from build123d import *

# Parameters (mm, degrees)
F0_R      = 174
F1_DEPTH  = 10
F2_R      = 5
F3_DEPTH  = 10
F4_R      = 5
F5_DEPTH  = 10
F6_R      = 10
F7_DEPTH  = 50
F9_R      = 9
F8_R      = 9
F10_R     = 9
F11_DEPTH = 60


with BuildPart() as f1:
    # F0 (on Top) → F1 (new body)
    with BuildSketch(Plane.XY):
        Circle(F0_R)
    extrude(amount=F1_DEPTH)

    # F2 (on face) → F3 (cut, through all)
    with BuildSketch(Plane.XY.offset(10)):
        with Locations((0, 160)):
            Circle(F2_R)
        with Locations((-113.137085, 113.137085)):
            Circle(F2_R)
        with Locations((-160, 0)):
            Circle(F2_R)
        with Locations((-113.137085, -113.137085)):
            Circle(F2_R)
        with Locations((0, -160)):
            Circle(F2_R)
        with Locations((113.137085, -113.137085)):
            Circle(F2_R)
        with Locations((160, 0)):
            Circle(F2_R)
        with Locations((113.137085, 113.137085)):
            Circle(F2_R)
    extrude(amount=-F3_DEPTH, mode=Mode.SUBTRACT)

    # F4 (on face) → F5 (cut, through all)
    with BuildSketch(Plane.XY.offset(10)):
        Circle(F4_R)
    extrude(amount=-F5_DEPTH, mode=Mode.SUBTRACT)

    # F6 (on face) → F7 (join)
    with BuildSketch(Plane.XY.offset(10)):
        with Locations((80, 0)):
            Circle(F6_R)
        with Locations((-40, 0)):
            Circle(F6_R)
        with Locations((-80, 0)):
            Circle(F6_R)
    extrude(amount=F7_DEPTH)

    # F9 (on face) + F8 (on face) + F10 (on face) → F11 (cut, through all)
    with BuildSketch(Plane.XY.offset(60)):
        with Locations((-80, 0)):
            Circle(F9_R)
    with BuildSketch(Plane.XY.offset(60)):
        with Locations((-40, 0)):
            Circle(F8_R)
    with BuildSketch(Plane.XY.offset(60)):
        with Locations((80, 0)):
            Circle(F10_R)
    extrude(amount=-F11_DEPTH, mode=Mode.SUBTRACT)


solid = f1.part
Check sheet for the modelled part. Datum: model origin and axes. Units: mm. A direction names the side the tool comes from. Round coordinates to 2 decimals unless told otherwise and drop trailing zeros. Order: outer loops, then holes, each group sorted by start corner. A loop starts at its lowest first (then second) coordinate and runs counter-clockwise, first axis right, second up. Notation, with made-up numbers: M 5,-13 L 47,-13 A22 ccw 47,16 Z; hole C -13,-9.75 d9. An arc over 180 degrees is marked long. One line per item, written item: value. Start each with the question number.
1. Section check A-A on z = 54.5. Enter the section's corners in (x, y).
2. Access from +Z, -Z, +X, -X, +Y, -Y to the whole of each face (thin tool, end or side, straight path). Record for faces 1 (the cylindrical face through (-50, 0, 35)), 2 (the cylindrical face through (155, 0, 5)).
3. Section check B-B on x = -80. Enter the section's corners in (y, z).
4. Scan lines: line 1 along Y through (x, z) = (-80, 22); line 2 along Z through (x, y) = (93.5, -121); line 3 along Y through (x, z) = (160, 8). Record each from-to range of solid material in increasing order.
5. Section check C-C on x = 0. Enter the section's corners in (y, z), and give its area (3 significant figures).
6. Gauge pin test, flat ends, axial feed: P1, Ø8, axis at x = -45, z = 11, coming from the +Y side; P2, Ø8, axis at x = -11.5, y = 22, coming from the +Z side; P3, Ø1, axis at x = -81.5, z = 18, coming from the +Y side. Record the tip position at first contact, or that the pin passes through.
7. Release check for a two-part mould opening along Y. For faces 3 (the flat face through (-89, 2, 60)), 4 (the cylindrical face through (2.307, 155.564, 5.07)), 5 (the cylindrical face through (-49, 0, 30)), 6 (the cylindrical face through (-90, 0, 35)) record: released by +Y, released by -Y, zero draft, split by the parting line, or undercut.
8. Section check D-D on y = 0. Give the number of separate pieces and of enclosed holes in the cut face, and give its area (3 significant figures).
Results found:
1. outline: C -80,0 d20; C -40,0 d20; C 80,0 d20; hole C -80,0 d18; hole C -40,0 d18; hole C 80,0 d18
2. face 1: +Z
2. face 2: +Z, -Z
3. outline: M -154.52,0 L -9,0 L -9,60 L -10,60 L -10,10 L -154.52,10 Z; M 9,0 L 154.52,0 L 154.52,10 L 10,10 L 10,60 L 9,60 Z
4. line 1: -10 to -9, 9 to 10
4. line 2: 0 to 10
4. line 3: -68.38 to -5, 5 to 68.38
5. outline: M -174,0 L -165,0 L -165,10 L -174,10 Z; M -155,0 L -5,0 L -5,10 L -155,10 Z; M 5,0 L 155,0 L 155,10 L 5,10 Z; M 165,0 L 174,0 L 174,10 L 165,10 Z
5. area: 3,180 mm^2
6. P1: y = 169.07
6. P2: z = 10
6. P3: y = 9.95
7. face 3: zero draft
7. face 4: undercut
7. face 5: undercut
7. face 6: split by the parting line
8. separate pieces: 7
8. enclosed holes: 0
8. area: 2,940 mm^2
